Input: part model. Units: mm. Frame: model coordinates. A direction names the side the tool comes from. Round coordinates to 2 decimals unless told otherwise and drop trailing zeros. Loops run counter-clockwise (first coordinate to the right, second up) from the corner with the lowest first, then second, coordinate; pieces in that order, holes last.
1) Ray query, line 1 along Y through (x, z) = (-3, 3.5); line 2 along Y through (x, z) = (0, -0.75); line 3 along X through (y, z) = (-21.5, 1.75). Return the intervals inside material, ascending.
2) First-contact query: pin 1 (1.5 mm diameter, centred on x = 2, z = 4.5, fed in from +Y); pin 2 (11 mm diameter, centred on x = -4.34, y = -17.34, fed in from -Z); pin 3 (1.1 mm diameter, centred on y = -25, z = -1.5, fed in from -X); pin 4 (6 mm diameter, centred on y = 33.5, z = 1.5, fed in from +X) (3 decimals). Flat tips, straight axial feed; report the tip coordinate or a pass-through.
3) Section B-B, the plane x = 4.5. Return loops of the section in (y, z), and give its area (3 significant figures).
4) Section A-A, the plane y = 0. Return loops of the section in (x, z).
5) Access query for faces 4 (the face through (0, 39.414, 0)), 5 (the face through (11, -11, 6.35)). Directions: +Z, -Z, +X, -X, +Y, -Y. A direction counts if a zero-diameter tool reaches every point of the face in a straight line with its end or side. Return the directions, or none.
6) Section C-C, the plane z = -4.25. Return loops of the section in (x, y) (3 decimals).
7) Section D-D, the plane x = 18.5. Return loops of the section in (y, z).
8) Draft query along X for faces 1 (the face through (-11.012, -49.592, 0.089)), 2 (the face through (11, -11, -6.35)), 3 (the face through (-1.775, -13.326, -0.089)). Return one class per face: pulls with the +X half, pulls with the -X half, needs draft (parallel to the pull), parting line crosses it, or undercut.
from build123d import *

# Parameters (mm, degrees)
F0_R     = 50.8
F0_R_2   = 4.7623858448
F0_R_3   = 12.7
F0_W     = 24.8306924477
F0_H     = 5.7149995118
F0_W_2   = 30.9398272075
F0_H_2   = 2.1677576005
F0_R_4   = 4.8592779804
F0_W_3   = 11.6270687431
F0_H_3   = 12.4153457582
F1_DEPTH = 6.35


# Not quite as in the source:
# - a length typed as a fraction of an inch, garbled in the dataset ("3 / 203.2 mm" for 3/8 in), is restored


with BuildPart() as f1:
    # F0 (on Top) → F1 (new body, symmetric)
    with BuildSketch(Plane.XY):
        Circle(F0_R)
        with Locations((-4.3355170637, -17.3420701176)):
            Circle(F0_R_2, mode=Mode.SUBTRACT)
        Circle(F0_R_3, mode=Mode.SUBTRACT)
        with Locations((7.6856906526, -32.2207761928)):
            Rectangle(F0_W, F0_H, mode=Mode.SUBTRACT)
        with Locations((7.7842238825, -25.3233611584)):
            Rectangle(F0_W_2, F0_H_2, mode=Mode.SUBTRACT)
        with Locations((15.0699028745, -17.0589182526)):
            Circle(F0_R_4, mode=Mode.SUBTRACT)
        with Locations((-0.0985348597, 33.206121996)):
            Rectangle(F0_W_3, F0_H_3, mode=Mode.SUBTRACT)
    extrude(amount=F1_DEPTH, both=True)


solid = f1.part
Final values:
1. line 1: y = -50.71 to -35.08, -29.36 to -26.41, -24.24 to -21.91, -12.77 to -12.34, 12.34 to 27, 39.41 to 50.71
1. line 2: y = -50.8 to -35.08, -29.36 to -26.41, -24.24 to -19.31, -15.37 to -12.7, 12.7 to 27, 39.41 to 50.8
1. line 3: x = -46.03 to -6.66, -2.01 to 13.1, 17.04 to 46.03
2. pin 1: stops at y = 50.78
2. pin 2: stops at z = -6.35
2. pin 3: stops at x = -44.53
2. pin 4: stops at x = 40.625
3. outline: (-50.6, -6.35) - (-35.08, -6.35) - (-35.08, 6.35) - (-50.6, 6.35) - close; (-29.36, -6.35) - (-26.41, -6.35) - (-26.41, 6.35) - (-29.36, 6.35) - close; (-24.24, -6.35) - (-11.88, -6.35) - (-11.88, 6.35) - (-24.24, 6.35) - close; (11.88, -6.35) - (27, -6.35) - (27, 6.35) - (11.88, 6.35) - close; (39.41, -6.35) - (50.6, -6.35) - (50.6, 6.35) - (39.41, 6.35) - close
3. area: 726 mm2
4. outline: (-50.8, -6.35) - (-12.7, -6.35) - (-12.7, 6.35) - (-50.8, 6.35) - close; (12.7, -6.35) - (50.8, -6.35) - (50.8, 6.35) - (12.7, 6.35) - close
5. face 4: +Z, -Z
5. face 5: +Z, +X, -X, +Y, -Y
6. outline: circle Ø101.6 at (0, 0); hole circle Ø25.4 at (0, 0); hole circle Ø9.525 at (-4.336, -17.342); hole (-7.686, -26.407) - (23.254, -26.407) - (23.254, -24.239) - (-7.686, -24.239) - close; hole (-5.912, 26.998) - (5.715, 26.998) - (5.715, 39.414) - (-5.912, 39.414) - close; hole (-4.73, -35.078) - (20.101, -35.078) - (20.101, -29.363) - (-4.73, -29.363) - close; hole circle Ø9.719 at (15.07, -17.059)
7. outline: (-47.31, -6.35) - (-35.08, -6.35) - (-35.08, 6.35) - (-47.31, 6.35) - close; (-29.36, -6.35) - (-26.41, -6.35) - (-26.41, 6.35) - (-29.36, 6.35) - close; (-24.24, -6.35) - (-20.5, -6.35) - (-20.5, 6.35) - (-24.24, 6.35) - close; (-13.62, -6.35) - (47.31, -6.35) - (47.31, 6.35) - (-13.62, 6.35) - close
8. face 1: parting line crosses it
8. face 2: needs draft
8. face 3: undercut
